```python
from build123d import *

# Parameters (mm, degrees)
F0_R     = 57.15
F0_R_2   = 50.8
F1_DEPTH = 1524
F2_W     = 127
F2_H     = 191.943108
F2_R     = 7.14375
F3_DEPTH = 6.35


with BuildPart() as f1:
    # F0 (on Top) → F1 (new body)
    with BuildSketch(Plane.XY):
        Circle(F0_R)
        Circle(F0_R_2, mode=Mode.SUBTRACT)
    extrude(amount=F1_DEPTH)

    # F2 (on face) → F3 (join)
    with BuildSketch(Plane.XY.offset(1524)):
        Rectangle(F2_W, F2_H)
        with Locations((-32.54375, -69.777804)):
            Circle(F2_R, mode=Mode.SUBTRACT)
        with Locations((32.54375, -69.777804)):
            Circle(F2_R, mode=Mode.SUBTRACT)
        with Locations((-32.54375, 69.777804)):
            Circle(F2_R, mode=Mode.SUBTRACT)
        with Locations((32.54375, 69.777804)):
            Circle(F2_R, mode=Mode.SUBTRACT)
    extrude(amount=F3_DEPTH)


solid = f1.part
```
Read the model definition and answer for the solid it produces. Units are mm, in the model's axes. A direction names the side the tool comes from. Round coordinates to 2 decimals unless told otherwise and drop trailing zeros. Write each loop counter-clockwise with the first axis right and the second up, starting at its lowest first coordinate (ties: lowest second). Pieces come first, ordered by that corner, then holes. Notation, with made-up numbers: (-26.75, 10) -> (-7.75, 10) arc R23 cw to (-7.75, 43) -> close; hole circle Ø2 at (-15.5, 76). An arc over 180 degrees is marked (long way). Answer in a Markdown table with one row per item. Add a question column.
1) Given P1, Ø18.5, axis at x = 32.54, y = 69.78, coming from the -Z side; P2, Ø8, axis at x = -38.5, z = 762.5, coming from the -Y side; P3, Ø3, axis at x = 30, z = 517.5, coming from the +Y side, each flat-ended and moving along its own axis, determine where each tip first touches the part or whether it passes through.
2) Consider line 1 (Y direction, x = 2, z = 937) (3 decimals); line 2 (Y direction, x = 4, z = 444.5); line 3 (Z direction, x = -19.5, y = 40.5). Determine where each line is inside the solid, lowest interval first.
3) Find section C-C, the plane z = 552.5. Determine the outline of the cut face in (x, y), and give its area (3 significant figures).
4) Which of the six approach directions +Z, -Z, +X, -X, +Y, -Y give full straight-line access (tool end or side, diameter ignored) to faces 1 (the face through (-57.3, 1.3, 1524)), 2 (the face through (-1, 1, 1530.35))?
5) Find section A-A, the plane y = 0. Determine the outline of the cut face in (x, z), and give its area (3 significant figures).
6) Find section B-B, the plane x = 0. Determine the outline of the cut face in (y, z).
7) Determine the mould class of faces 3 (the face through (-57.095, 2.513, 751.332)), 4 (the face through (-11.012, -49.592, 751.332)), 5 (the face through (-38, -34, 0)) for opening direction X: pulls with the +X half, pulls with the -X half, needs draft (parallel to the pull), parting line crosses it, or undercut.
Findings below:
| question | item | result |
|---|---|---|
| 1 | P1 | z = 1524 |
| 1 | P2 | y = -45.56 |
| 1 | P3 | y = 49.54 |
| 2 | line 1 | -57.115 to -50.761, 50.761 to 57.115 |
| 2 | line 2 | -57.01 to -50.64, 50.64 to 57.01 |
| 2 | line 3 | 1524 to 1530.35 |
| 3 | outline | circle Ø114.3 at (0, 0); hole circle Ø101.6 at (0, 0) |
| 3 | area | 2,150 mm² |
| 4 | face 1 | -Z |
| 4 | face 2 | +Z, +X, -X, +Y, -Y |
| 5 | outline | (-63.5, 1524) -> (-57.15, 1524) -> (-57.15, 0) -> (-50.8, 0) -> (-50.8, 1524) -> (50.8, 1524) -> (50.8, 0) -> (57.15, 0) -> (57.15, 1524) -> (63.5, 1524) -> (63.5, 1530.35) -> (-63.5, 1530.35) -> close |
| 5 | area | 20,200 mm² |
| 6 | outline | (-95.97, 1524) -> (-57.15, 1524) -> (-57.15, 0) -> (-50.8, 0) -> (-50.8, 1524) -> (50.8, 1524) -> (50.8, 0) -> (57.15, 0) -> (57.15, 1524) -> (95.97, 1524) -> (95.97, 1530.35) -> (-95.97, 1530.35) -> close |
| 7 | face 3 | parting line crosses it |
| 7 | face 4 | undercut |
| 7 | face 5 | needs draft |
